Source: three-view drawing plus pictorial views. Frame: mm from the lowest corner of the part. A direction names the side the tool comes from. Coordinates: 2 decimals unless noted, no trailing zeros. Write each loop counter-clockwise with the first axis right and the second up, starting at its lowest first coordinate (ties: lowest second). Pieces come first, ordered by that corner, then holes. Notation, with made-up numbers: (68.25, -19) -> (118.25, -19) arc R15 ccw to (118.25, -6) -> close; hole circle Ø7 at (-30.5, -39). An arc over 180 degrees is marked (long way). One line per item, written item: value. Start each with the question number.
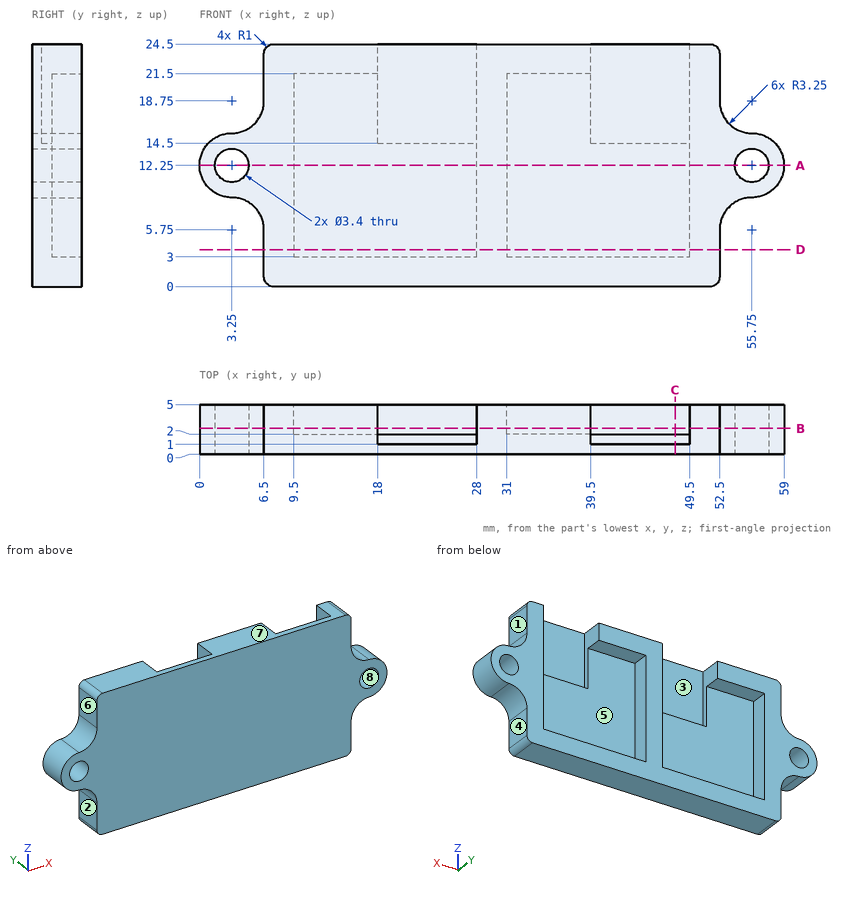
Q1. Draft query along X for the marked faces 6, 7 and 8. Return one class per face: pulls with the +X half, pulls with the -X half, needs draft (parallel to the pull), parting line crosses it, or undercut.
Q2. First-contact query: P1, Ø2, axis at y = 3, z = 21, coming from the -X side; P2, Ø1.5, axis at y = 4, z = 8, coming from the +X side; P3, Ø2.5, axis at y = 3.5, z = 10.5, coming from the +X side; P4, Ø2, axis at x = 3.25, z = 12.25, coming from the +Y side. Flat tips, straight axial feed; report the tip coordinate or a pass-through.
Q3. Line query: L1, parallel to X at y = 2.05, z = 5.5; L2, parallel to X at y = 3, z = 12.25; L3, parallel to X at y = 4.7, z = 22. Output: solid intervals per line, ascending. Write a range as from..to.
Q4. Access query for the marked faces 1, 2, 3, 4 and 5. Directions: +Z, -Z, +X, -X, +Y, -Y. A direction counts if a zero-diameter tool reaches every point of the face in a straight line with its end or side. Return the directions, or none.
Q5. Cut plane B-B on y = 2.6. Count the separate pieces of the cut face and the enclosed holes in it, and give its area (3 significant figures).
Q6. Cut plane C-C on x = 48. Output: boundary loops of the cut face in (y, z).
Q7. Cut plane A-A on z = 12.25. Output: boundary loops of the cut face in (x, y).
Q8. Cut plane D-D on z = 3.75. Output: boundary loops of the cut face in (x, y).
Solution:
1. face 6: pulls with the -X half
1. face 7: needs draft
1. face 8: undercut
2. P1: x = 6.5
2. P2: x = 54.5
2. P3: x = 58.96
2. P4: through
3. L1: 6.5..9.5, 28..31, 49.5..52.5
3. L2: 0..1.55, 4.95..9.5, 28..31, 49.5..54.05, 57.45..59
3. L3: 6.5..18, 28..39.5, 49.5..52.5
4. face 1: +Z, +X, +Y, -Y
4. face 2: -Z, -X, +Y, -Y
4. face 3: +Z, +Y
4. face 4: -Z, +X, +Y, -Y
4. face 5: +Y
5. separate pieces: 1
5. enclosed holes: 2
5. area: 448 mm²
6. outline: (0, 0) -> (5, 0) -> (5, 3) -> (2, 3) -> (2, 14.5) -> (1, 14.5) -> (1, 24.5) -> (0, 24.5) -> close
7. outline: (0, 0) -> (1.55, 0) -> (1.55, 5) -> (0, 5) -> close; (4.95, 0) -> (54.05, 0) -> (54.05, 5) -> (49.5, 5) -> (49.5, 2) -> (31, 2) -> (31, 5) -> (28, 5) -> (28, 2) -> (9.5, 2) -> (9.5, 5) -> (4.95, 5) -> close; (57.45, 0) -> (59, 0) -> (59, 5) -> (57.45, 5) -> close
8. outline: (6.5, 0) -> (52.5, 0) -> (52.5, 5) -> (49.5, 5) -> (49.5, 2) -> (31, 2) -> (31, 5) -> (28, 5) -> (28, 2) -> (9.5, 2) -> (9.5, 5) -> (6.5, 5) -> close
